Can you work these out from the drawing? Everything is in mm from the part's minimum corner. A direction names the side the tool comes from. Give positions to 0.01 mm unless a question says otherwise; leave off trailing zeros. Write each loop counter-clockwise with the first axis right and the second up, starting at its lowest first coordinate (ties: lowest second). Pieces come first, ordered by that corner, then holes. Notation, with made-up numbers: (18.5, 75) - (31.5, 75) arc R29 ccw to (31.5, 102) - close; hole circle Ø7 at (0, 73.5). An arc over 180 degrees is marked (long way). Use a Markdown table: item, result. Add a question column.
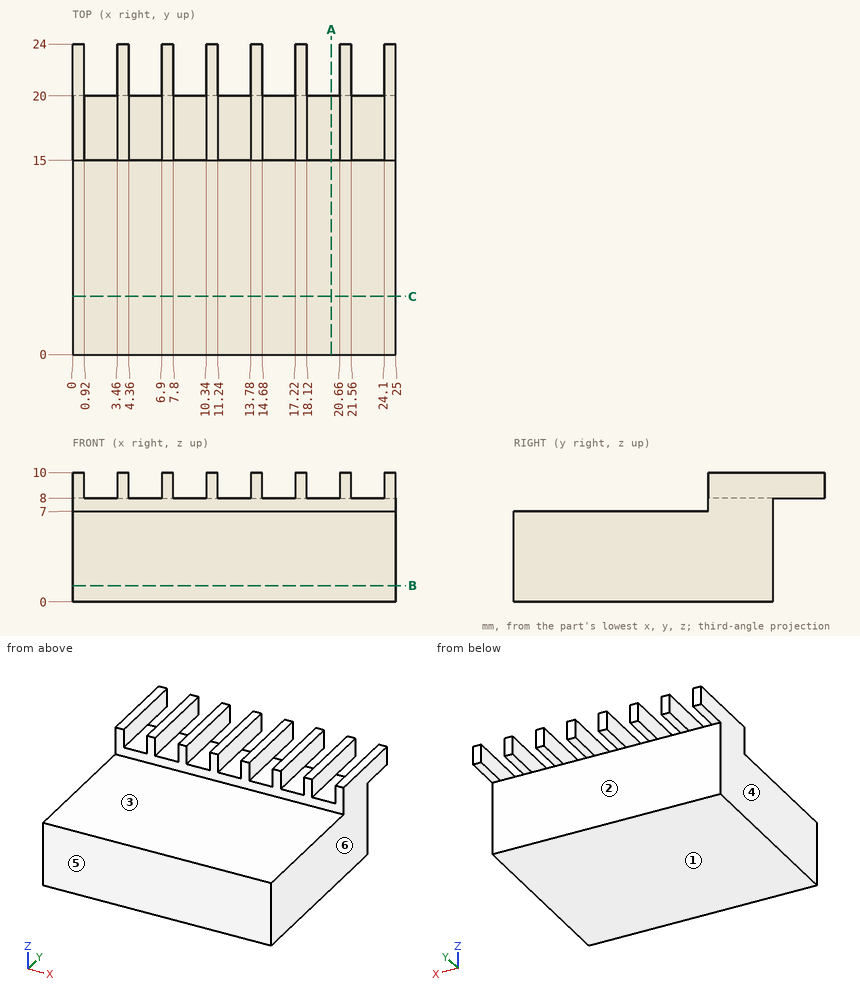
Q1. Suppose I cut it at A-A (x = 20). Please give me the cut outline in (y, z), and give its area (3 significant figures).
Q2. I'm going to push flat-ended pins straight in: P1, Ø2, axis at x = 9, y = 16.5, coming from the +Z side; P2, Ø0.7, axis at x = 24.5, y = 22, coming from the -Z side; P3, Ø1.6, axis at y = 17.5, z = 8.5, coming from the -X side; P4, Ø4, axis at x = 20, y = 8.5, coming from the +Z side. Where does each tip first touch, or does it pass through?
Q3. Suppose I cut it at C-C (y = 4.5). Please give me the cut outline in (x, z), and give its area (3 significant figures).
Q4. On a 3-axis mill with a long thin cutter (end or side, diameter ignored), from which of +Z, -Z, +X, -X, +Y, -Y can I reach the whole of each face in a straight line? I mean the marked faces 1, 2 and 3. Say none if no direction works.
Q5. If we mould it in two halves opening along X, with no side actions, what happens to the marked faces 4, 5 and 6? For each: released by +X, released by -X, zero draft, split by the parting line, or undercut.
Q6. If I drill on probe 1 along Y at (x, z) = (1.5, 6.75); probe 2 along Z at (x, y) = (23.5, 12.5); probe 3 along Z at (x, y) = (19, 19.25), over which ranges is the centre line in solid material (lowest first)? Write a range as [from, to].
Q7. Suppose I cut it at B-B (z = 1.25). Please give me the cut outline in (x, y).
Derived:
| question | item | result |
|---|---|---|
| 1 | outline | (0, 0) - (20, 0) - (20, 8) - (15, 8) - (15, 7) - (0, 7) - close |
| 1 | area | 145 mm² |
| 2 | P1 | z = 8 |
| 2 | P2 | z = 8 |
| 2 | P3 | x = 0 |
| 2 | P4 | z = 7 |
| 3 | outline | (0, 0) - (25, 0) - (25, 7) - (0, 7) - close |
| 3 | area | 175 mm² |
| 4 | face 1 | -Z, +X, -X, +Y, -Y |
| 4 | face 2 | -Z, +X, -X, +Y |
| 4 | face 3 | +Z, +X, -X, -Y |
| 5 | face 4 | released by -X |
| 5 | face 5 | zero draft |
| 5 | face 6 | released by +X |
| 6 | probe 1 | [0, 20] |
| 6 | probe 2 | [0, 7] |
| 6 | probe 3 | [0, 8] |
| 7 | outline | (0, 0) - (25, 0) - (25, 20) - (0, 20) - close |
